Autodesk Inventor part; units mm, degrees
ref_plane "YZ Plane" through (0, 0, 0) normal (1, 0, 0) x (0, 1, 0)
ref_plane "XZ Plane" through (0, 0, 0) normal (0, 1, 0) x (-1, 0, 0)
ref_plane "XY Plane" through (0, 0, 0) normal (0, 0, 1) x (1, 0, 0)
sketch "Sketch1" plane through (0, 0, 0) normal (0, 1, 0) x (-1, 0, 0)
  line L0 (13.85, 27.5) -> (-13.85, 27.5)
  line L1 (-13.85, 27.5) -> (-13.85, -27.5)
  line L2 (-13.85, -27.5) -> (13.85, -27.5)
  line L3 (13.85, -27.5) -> (13.85, 27.5)
  line L4 (13.85, 27.5) -> (-13.85, -27.5) construction
  line L5 (-13.85, 27.5) -> (13.85, -27.5) construction
  line L6 (0, 27.5) -> (0, -27.5) construction
  line L7 (13.85, 0) -> (-13.85, 0) construction
  circle A0 centre (11.51, 25.4) radius 1.5
  circle A1 centre (11.51, -25.4) radius 1.5
  circle A2 centre (-11.51, 25.4) radius 1.5
  circle A3 centre (-11.51, -25.4) radius 1.5
  point P0 (0, 0)
  dimension "d0" = 27.7
  dimension "d1" = 55
  dimension "d2" = 3
  dimension "d3" = 2.34
  dimension "d4" = 2.1
extrude "Extrusion1" add sketch "Sketch1" along normal blind 1
properties part number "esp32_footprint"
Geometry: final body of the model. Coordinates: model frame, mm. Coordinates: 2 decimals unless noted, no trailing zeros. Loops run counter-clockwise (first coordinate to the right, second up) from the corner with the lowest first, then second, coordinate; pieces in that order, holes last. Notation, with made-up numbers: M 72.5,52 L 130.5,52 A27 cw 130.5,76 Z; hole C -26.75,-4.75 d11. An arc over 180 degrees is marked long. One line per item, written item: value. Start each with the question number.
1) Cut plane B-B (x = 11.51). Return loops of the section in (y, z).
2) Cut plane A-A (z = 25.4). Return loops of the section in (x, y), then the cut area to 3 significant figures.
3) Cut plane C-C (y = 0.35). Return loops of the section in (x, z).
4) Draft query along Z for faces 1 (the cylindrical face through (12.62, 0.49, 24.39)), 2 (the flat face through (0, 0, 0)), 3 (the cylindrical face through (-10.32, 0.49, -24.49)), 4 (the flat face through (0.2, 0.5, -27.5)). Return one class per face: released by +Z, released by -Z, zero draft, split by the parting line, or undercut.
5) Material intervals for L1, parallel to Z at x = 11.51, y = 0.2; L2, parallel to Z at x = 12.75, y = 0.3, sorted ascending. Write a range as from..to.
Evaluation:
1. outline: M 0,-27.5 L 1,-27.5 L 1,-26.9 L 0,-26.9 Z; M 0,-23.9 L 1,-23.9 L 1,23.9 L 0,23.9 Z; M 0,26.9 L 1,26.9 L 1,27.5 L 0,27.5 Z
2. outline: M -13.85,0 L -13.01,0 L -13.01,1 L -13.85,1 Z; M -10.01,0 L 10.01,0 L 10.01,1 L -10.01,1 Z; M 13.01,0 L 13.85,0 L 13.85,1 L 13.01,1 Z
2. area: 21.7 mm^2
3. outline: M -13.85,-27.5 L 13.85,-27.5 L 13.85,27.5 L -13.85,27.5 Z; hole C -11.51,-25.4 d3; hole C -11.51,25.4 d3; hole C 11.51,-25.4 d3; hole C 11.51,25.4 d3
4. face 1: undercut
4. face 2: zero draft
4. face 3: undercut
4. face 4: released by -Z
5. L1: -27.5..-26.9, -23.9..23.9, 26.9..27.5
5. L2: -27.5..-26.24, -24.56..24.56, 26.24..27.5
